Verification items for the finished model (mm, model axes). Face numbers are marked on the shaded views. A direction names the side the tool comes from. Round coordinates to 2 decimals unless told otherwise and drop trailing zeros. Loops run counter-clockwise (first coordinate to the right, second up) from the corner with the lowest first, then second, coordinate; pieces in that order, holes last. Notation, with made-up numbers: (-36.75, 68) - (-2.75, 68) arc R24 cw to (-2.75, 85) - close; hole circle Ø1 at (-14, 86). An arc over 180 degrees is marked (long way). Use CSV: the item, a comma, the result in double quotes.
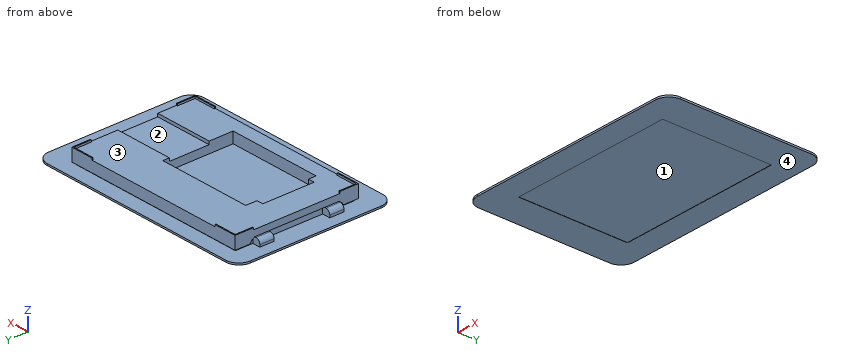
```python
from build123d import *

# Parameters (mm, degrees)
CROQUIS1_W              = 85
CROQUIS1_H              = 56.6
SALIENTE_EXTRUIR1_DEPTH = 5
SALIENTE_EXTRUIR2_DEPTH = 0.85
CROQUIS3_W              = 83
CROQUIS3_H              = 54.6
SALIENTE_EXTRUIR3_DEPTH = 0.9
SALIENTE_EXTRUIR4_DEPTH = 0.8
CROQUIS5_W              = 75
CROQUIS5_H              = 50
CORTAR_EXTRUIR1_DEPTH   = 0.1
CROQUIS6_W              = 26.8
CROQUIS6_H              = 18.3
CORTAR_EXTRUIR2_DEPTH   = 1.4
CROQUIS7_W              = 2.1
CROQUIS7_H              = 42.6
CORTAR_EXTRUIR3_DEPTH   = 1
REDONDEO1_R             = 2.9
SALIENTE_EXTRUIR5_REACH = 117.643
CROQUIS8_W              = 3.7
CROQUIS8_H              = 6.5
REDONDEO2_R             = 2


with BuildPart() as part:
    # Croquis1 → Saliente-Extruir1 (new body)
    with BuildSketch(Plane.XY):
        with Locations((42.5, 28.3)):
            Rectangle(CROQUIS1_W, CROQUIS1_H)
        Polygon((12, 33.3), (12, 9.7), (15, 9.7), (15, 6.2), (58.2, 6.2), (58.2, 38.5), (15, 38.5), (15, 33.3), align=None, mode=Mode.SUBTRACT)
    extrude(amount=SALIENTE_EXTRUIR1_DEPTH)

    # Croquis2 → Saliente-Extruir2 (add)
    with BuildSketch(Plane.XY.offset(5)):
        Polygon((0, 56.6), (10.5, 56.6), (10.5, 56.1), (0.5, 56.1), (0.5, 48.1), (0, 48.1), align=None)
        Polygon((85, 48.1), (85, 56.6), (74.5, 56.6), (74.5, 56.1), (84.5, 56.1), (84.5, 48.1), align=None)
        Polygon((85, 0), (74.5, 0), (74.5, 0.5), (84.5, 0.5), (84.5, 8.5), (85, 8.5), align=None)
        Polygon((0, 8.5), (0, 0), (10.5, 0), (10.5, 0.5), (0.5, 0.5), (0.5, 8.5), align=None)
    extrude(amount=SALIENTE_EXTRUIR2_DEPTH)

    # Croquis3 → Saliente-Extruir3 (add)
    with BuildSketch(Plane(origin=(0, 0, 0), x_dir=(-1, 0, 0), z_dir=(0, 0, -1))):
        with Locations((-42.5, 28.3)):
            Rectangle(CROQUIS3_W, CROQUIS3_H)
    extrude(amount=SALIENTE_EXTRUIR3_DEPTH)

    # Croquis4 → Saliente-Extruir4 (add)
    with BuildSketch(Plane(origin=(0, 0, -0.9), x_dir=(-1, 0, 0), z_dir=(0, 0, -1))):
        with BuildLine():
            Line((-91, 62.6), (2, 62.6))
            ThreePointArc((2, 62.6), (6.242640687, 60.842640687), (8, 56.6))
            Line((8, 56.6), (8, -3.4))
            ThreePointArc((8, -3.4), (6.242640687, -7.642640687), (2, -9.4))
            Line((2, -9.4), (-91, -9.4))
            ThreePointArc((-91, -9.4), (-95.242640687, -7.642640687), (-97, -3.4))
            Line((-97, -3.4), (-97, 56.6))
            ThreePointArc((-97, 56.6), (-95.242640687, 60.842640687), (-91, 62.6))
        make_face()
    extrude(amount=SALIENTE_EXTRUIR4_DEPTH)

    # Croquis5 → Cortar-Extruir1 (cut)
    with BuildSketch(Plane(origin=(0, 0, -1.7), x_dir=(-1, 0, 0), z_dir=(0, 0, -1))):
        with Locations((-44.5, 26.6)):
            Rectangle(CROQUIS5_W, CROQUIS5_H)
    extrude(amount=-CORTAR_EXTRUIR1_DEPTH, mode=Mode.SUBTRACT)

    # Croquis6 → Cortar-Extruir2 (cut)
    with BuildSketch(Plane.XY.offset(5)):
        with Locations((71.6, 26.35)):
            Rectangle(CROQUIS6_W, CROQUIS6_H)
    extrude(amount=-CORTAR_EXTRUIR2_DEPTH, mode=Mode.SUBTRACT)

    # Croquis7 → Cortar-Extruir3 (cut)
    with BuildSketch(Plane.ZY):
        with Locations((1.05, 28.3)):
            Rectangle(CROQUIS7_W, CROQUIS7_H)
    extrude(amount=-CORTAR_EXTRUIR3_DEPTH, mode=Mode.SUBTRACT)

    # Redondeo1
    # the kernel refuses this fillet: 2.9 mm, written as the material it adds along each edge
    with BuildSketch(Plane(origin=(0, 7, 2.1), x_dir=(0, 0, -1), z_dir=(1, 0, 0))) as redondeo1_piece_1:
        with BuildLine():
            CenterArc((2.9, 2.787471973), REDONDEO1_R, 180, 73.986605576)
            Line((0, 2.787471973), (-0.058, 2.787471973))
            Line((-0.058, 2.787471973), (-0.058, 0))
            Line((-0.058, 0), (0, -0.058))
            ThreePointArc((0, -0.058), (1.05, -0.058), (2.084, -0.055749439))
            Line((2.084, -0.055749439), (2.1, 0))
        make_face()
    extrude(amount=7.968679932)
    with BuildSketch(Plane(origin=(0, 49.6, 2.1), x_dir=(0, 0, -1), z_dir=(1, 0, 0))) as redondeo1_piece_2:
        with BuildLine():
            CenterArc((2.9, -2.787471973), REDONDEO1_R, 106.013394424, 73.986605576)
            Line((0, -2.787471973), (-0.058, -2.787471973))
            Line((-0.058, -2.787471973), (-0.058, 0))
            Line((-0.058, 0), (0, 0.058))
            ThreePointArc((0, 0.058), (1.05, 0.058), (2.084, 0.055749439))
            Line((2.084, 0.055749439), (2.1, 0))
        make_face()
    extrude(amount=7.968679932)

    # Saliente-Extruir5: up to this face of the body (flat: up to its plane)
    saliente_extruir5_end = Plane(part.part.faces().sort_by_distance((0.5, 28.3, 2.1))[0])
    # Croquis8 → Saliente-Extruir5 (add, up to the picked face)
    with BuildSketch(Plane.XY.offset(-0.9), mode=Mode.PRIVATE) as saliente_extruir5_sk1:
        with Locations((-0.85, 44.35)):
            Rectangle(CROQUIS8_W, CROQUIS8_H)
    saliente_extruir5_tool1 = split(extrude(saliente_extruir5_sk1.sketch, amount=SALIENTE_EXTRUIR5_REACH, mode=Mode.PRIVATE), bisect_by=saliente_extruir5_end, keep=Keep.BOTH, mode=Mode.PRIVATE)
    # Croquis8 → Saliente-Extruir5 (add, up to the picked face)
    with BuildSketch(Plane.XY.offset(-0.9), mode=Mode.PRIVATE) as saliente_extruir5_sk2:
        with Locations((-0.85, 12.25)):
            Rectangle(CROQUIS8_W, CROQUIS8_H)
    saliente_extruir5_tool2 = split(extrude(saliente_extruir5_sk2.sketch, amount=SALIENTE_EXTRUIR5_REACH, mode=Mode.PRIVATE), bisect_by=saliente_extruir5_end, keep=Keep.BOTH, mode=Mode.PRIVATE)
    add(saliente_extruir5_tool1.solids().sort_by(Axis((-0.85, 44.35, -0.9), (0, 0, 1)))[0])
    add(saliente_extruir5_tool2.solids().sort_by(Axis((-0.85, 12.25, -0.9), (0, 0, 1)))[0])

    # Redondeo2
    redondeo2_edges = [part.edges().sort_by_distance(p)[0] for p in [
        (-2.7, 44.35, 2.1),
        (-2.7, 12.25, 2.1),
    ]]
    fillet(redondeo2_edges, radius=REDONDEO2_R)


solid = part.part
```
1) Access from +Z, -Z, +X, -X, +Y, -Y to the whole of each face (thin tool, end or side, straight path). Record for the marked faces 1 and 2.
Returned:
face 1,"-Z"
face 2,"+Z, +X"
2) Thickness scan on probe 1 along Y at (x, z) = (58, 3.5); probe 2 along X at (y, z) = (18, 3); probe 3 along Y at (x, z) = (62, 4.25). Record the ranges inside material, lowest first. Write a range as [from, to].
Returned:
probe 1,"y = [0, 6.2], [38.5, 56.6]"
probe 2,"x = [0, 12], [58.2, 85]"
probe 3,"y = [0, 17.2], [35.5, 56.6]"
3) Cross-section at C-C, the plane x = 88. Record the cut outline in (y, z).
Returned:
outline,"(-9.4, -1.7) - (62.6, -1.7) - (62.6, -0.9) - (-9.4, -0.9) - close"
4) Cross-section at B-B, the plane x = 39. Record the cut outline in (y, z).
Returned:
outline,"(-9.4, -1.7) - (1.6, -1.7) - (1.6, -1.6) - (51.6, -1.6) - (51.6, -1.7) - (62.6, -1.7) - (62.6, -0.9) - (55.6, -0.9) - (55.6, 0) - (56.6, 0) - (56.6, 5) - (38.5, 5) - (38.5, 0) - (6.2, 0) - (6.2, 5) - (0, 5) - (0, 0) - (1, 0) - (1, -0.9) - (-9.4, -0.9) - close"
5) Mould release check, pull along Y, two halves, no side actions. Record for the marked faces 3 and 4: +Y half, -Y half, draft (parallel to the pull), parting line (faces both ways), or undercut.
Returned:
face 3,"undercut"
face 4,"draft"
6) Cross-section at A-A, the plane y = 32. Record the cut outline in (x, z).
Returned:
outline,"(-8, -1.7) - (7, -1.7) - (7, -1.6) - (82, -1.6) - (82, -1.7) - (97, -1.7) - (97, -0.9) - (84, -0.9) - (84, 0) - (85, 0) - (85, 3.6) - (58.2, 3.6) - (58.2, 0) - (12, 0) - (12, 5) - (0, 5) - (0, 2.1) - (1, 2.1) - (1, -0.9) - (-8, -0.9) - close"
7) Gauge pin test, flat ends, axial feed: pin 1 Ø1.5 at (x, z) = (29, 3.5) entering from -Y; pin 2 Ø1 at (y, z) = (8, 2) entering from +X; pin 3 Ø2.5 at (x, z) = (45, 3.5) entering from +Y. Record the tip position at first contact, or that the pin passes through.
Returned:
pin 1,"stops at y = 0"
pin 2,"stops at x = 85"
pin 3,"stops at y = 56.6"
